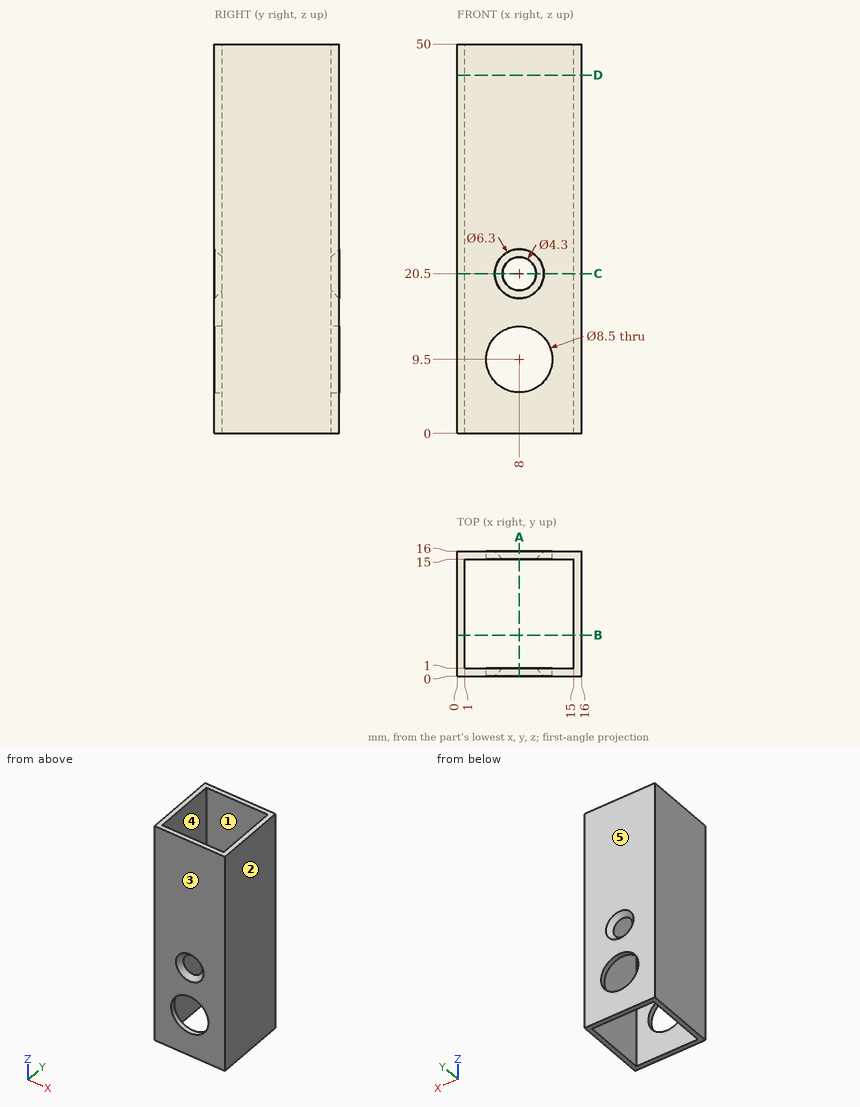
Design review of the part shown in the three views and the two pictorial views. Dimensions are in mm from the part's minimum x, y and z. A direction names the side the tool comes from. Give positions to 0.01 mm unless a question says otherwise; leave off trailing zeros. Write each loop counter-clockwise with the first axis right and the second up, starting at its lowest first coordinate (ties: lowest second). Pieces come first, ordered by that corner, then holes. Notation, with made-up numbers: (26, 64) - (43, 64) arc R5 cw to (43, 73) - close; hole circle Ø7 at (16, 80.5). An arc over 180 degrees is marked (long way). Return JSON: item names as keys, results as strings. Group by question number.
(1) Insertion check: pin 1 (1.5 mm diameter, centred on x = 12, z = 12.5, fed in from -Y). The pin has a flat end and moves straight along its axis. Give the tip position at first contact, or say it passes through.
(2) Machinability: for the marked faces 4 and 5, which of the approach directions +Z, -Z, +X, -X, +Y, -Y give a long, thin tool a straight path to every point of the face, cutting with its end or side? Answer none if there is none.
(3) We need section A-A, the plane x = 8. Give the boundary of the cut face in (y, z), then the cut area to 3 significant figures.
(4) To check wall thickness, follow probe 1 along Y at (x, z) = (2.25, 9.5); probe 2 along X at (y, z) = (15.45, 9.5). State the ranges of each line that lie inside material, in increasing order.
(5) We need section B-B, the plane y = 5.25. Give the boundary of the cut face in (x, z).
(6) We need section D-D, the plane z = 46. Give the boundary of the cut face in (x, y), then the cut area to 3 significant figures.
(7) Mouldability with a two-part tool opening along X and no side actions: class the marked faces 1, 2 and 3 as +X half, -X half, draft (parallel to the pull), parting line (faces both ways), or undercut.
(8) We need section C-C, the plane z = 20.5. Give the boundary of the cut face in (x, y), then the cut area to 3 significant figures.
Reported:
{
 "1": {"pin 1": "stops at y = 0"},
 "2": {"face 4": "+Z, -Z", "face 5": "+Z, -Z, +X, -X, +Y"},
 "3": {"outline": "(0, 0) - (1, 0) - (1, 5.25) - (0, 5.25) - close; (0, 13.75) - (1, 13.75) - (1, 18.35) - (0, 17.35) - close; (0, 23.65) - (1, 22.65) - (1, 50) - (0, 50) - close; (15, 0) - (16, 0) - (16, 5.25) - (15, 5.25) - close; (15, 13.75) - (16, 13.75) - (16, 17.35) - (15, 18.35) - close; (15, 22.65) - (16, 23.65) - (16, 50) - (15, 50) - close", "area": "72.4 mm2"},
 "4": {"probe 1": "y = 0 to 1, 15 to 16", "probe 2": "x = 0 to 3.75, 12.25 to 16"},
 "5": {"outline": "(0, 0) - (1, 0) - (1, 50) - (0, 50) - close; (15, 0) - (16, 0) - (16, 50) - (15, 50) - close"},
 "6": {"outline": "(0, 0) - (16, 0) - (16, 16) - (0, 16) - close; hole (1, 1) - (15, 1) - (15, 15) - (1, 15) - close", "area": "60.0 mm2"},
 "7": {"face 1": "undercut", "face 2": "+X half", "face 3": "draft"},
 "8": {"outline": "(0, 0) - (4.85, 0) - (5.85, 1) - (1, 1) - (1, 15) - (5.85, 15) - (4.85, 16) - (0, 16) - close; (10.15, 1) - (11.15, 0) - (16, 0) - (16, 16) - (11.15, 16) - (10.15, 15) - (15, 15) - (15, 1) - close", "area": "49.4 mm2"}
}
